Check sheet for the drawn part. Datum: minimum x, y, z corner. Units: mm. Round coordinates to 2 decimals unless told otherwise and drop trailing zeros. Write each loop counter-clockwise with the first axis right and the second up, starting at its lowest first coordinate (ties: lowest second). Pieces come first, ordered by that corner, then holes. Notation, with made-up numbers: M -28.75,-29.75 L 1.25,-29.75 A20 cw 1.25,-13.75 Z; hole C -27,-5 d8. An arc over 180 degrees is marked long. Use a Markdown table: item, result.
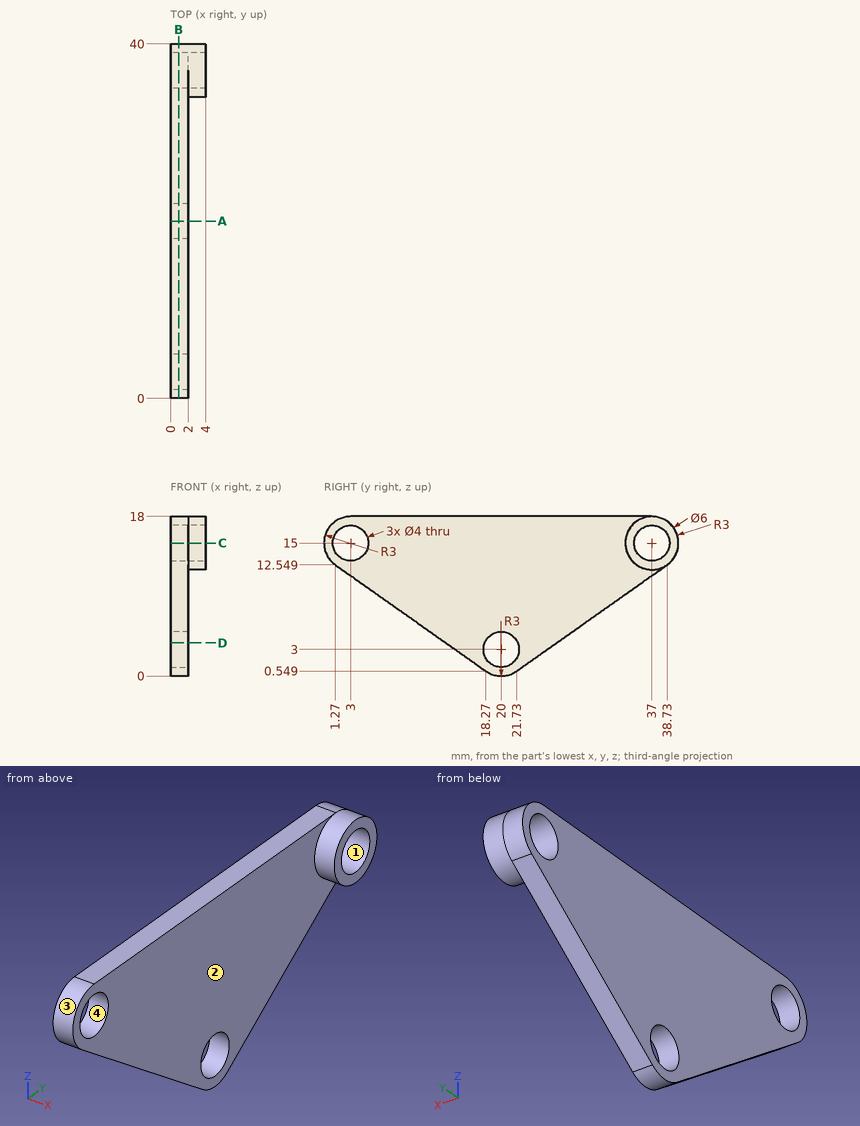
Item 1: Cross-section at B-B, the plane x = 0.9. Record the cut outline in (y, z), and give its area (3 significant figures).
Outcome:
| item | result |
|---|---|
| outline | M 1.27,12.55 L 18.27,0.55 A3 ccw 21.73,0.55 L 38.73,12.55 A3 ccw 37,18 L 3,18 A3 ccw Z; hole C 3,15 d4; hole C 20,3 d4; hole C 37,15 d4 |
| area | 421 mm2 |
Item 2: Material ranges on line 1 along Y through (x, z) = (0.55, 15); line 2 along Z through (x, y) = (1.35, 20); line 3 along Y through (x, z) = (3.05, 15), recorded low to high. Write a range as from..to.
Outcome:
| item | result |
|---|---|
| line 1 | y = 0..1, 5..35, 39..40 |
| line 2 | z = 0..1, 5..18 |
| line 3 | y = 34..35, 39..40 |
Item 3: Go/stop test with a flat-tipped pin: pin 1 (1 mm diameter, centred on x = 0.5, z = 14, fed in from +Y). Record where the tip stops, or that it passes through.
Outcome:
| item | result |
|---|---|
| pin 1 | stops at y = 39.96 |
Item 4: Cross-section at A-A, the plane y = 20. Record the cut outline in (x, z), and give its area (3 significant figures).
Outcome:
| item | result |
|---|---|
| outline | M 0,0 L 2,0 L 2,1 L 0,1 Z; M 0,5 L 2,5 L 2,18 L 0,18 Z |
| area | 28.0 mm2 |
Item 5: Mould release check, pull along Y, two halves, no side actions. Record for the marked faces 1, 2, 3 and 4: +Y half, -Y half, draft (parallel to the pull), parting line (faces both ways), or undercut.
Outcome:
| item | result |
|---|---|
| face 1 | undercut |
| face 2 | draft |
| face 3 | -Y half |
| face 4 | undercut |
Item 6: Cross-section at C-C, the plane z = 15. Record the cut outline in (x, y).
Outcome:
| item | result |
|---|---|
| outline | M 0,0 L 2,0 L 2,1 L 0,1 Z; M 0,5 L 2,5 L 2,34 L 4,34 L 4,35 L 0,35 Z; M 0,39 L 4,39 L 4,40 L 0,40 Z |
Item 7: Cross-section at D-D, the plane z = 3.75. Record the cut outline in (x, y).
Outcome:
| item | result |
|---|---|
| outline | M 0,13.74 L 2,13.74 L 2,18.15 L 0,18.15 Z; M 0,21.85 L 2,21.85 L 2,26.26 L 0,26.26 Z |
